```python
from build123d import *

# Parameters (mm, degrees)
SKETCH_1_W          = 49
SKETCH_1_H          = 34.996183206
EXTRUDE_1_DEPTH     = 3
CHAMFER_1_SIZE      = 9.5
FILLET_1_R          = 3
SKETCH_2_R          = 1.65
CUT_EXTRUDE_1_DEPTH = 4


with BuildPart() as part:
    # 草图1 → 凸台-拉伸1 (new body)
    with BuildSketch(Plane.XY):
        Rectangle(SKETCH_1_W, SKETCH_1_H)
    extrude(amount=EXTRUDE_1_DEPTH)

    # 倒角1
    chamfer_1_edges = [part.edges().sort_by_distance(p)[0] for p in [
        (24.5, -17.498091603, 1.5),
        (-24.5, -17.498091603, 1.5),
        (-24.5, 17.498091603, 1.5),
        (24.5, 17.498091603, 1.5),
    ]]
    chamfer(chamfer_1_edges, length=CHAMFER_1_SIZE)

    # 圆角1
    fillet_1_edges = [part.edges().sort_by_distance(p)[0] for p in [
        (-24.5, -7.998091603, 1.5),
        (-24.5, 7.998091603, 1.5),
        (15, 17.498091603, 1.5),
        (-15, 17.498091603, 1.5),
        (15, -17.498091603, 1.5),
        (-15, -17.498091603, 1.5),
        (24.5, 7.998091603, 1.5),
        (24.5, -7.998091603, 1.5),
    ]]
    fillet(fillet_1_edges, radius=FILLET_1_R)

    # 草图2 → 切除-拉伸1 (cut, through all)
    with BuildSketch(Plane.XY.offset(3)):
        with Locations((-21.5, 0)):
            Circle(SKETCH_2_R)
        with Locations((21.5, 0)):
            Circle(SKETCH_2_R)
    extrude(amount=-CUT_EXTRUDE_1_DEPTH, mode=Mode.SUBTRACT)


solid = part.part
```
Verification items for the finished model (mm, model axes). Coordinates: 2 decimals unless noted, no trailing zeros. Write each loop counter-clockwise with the first axis right and the second up, starting at its lowest first coordinate (ties: lowest second). Pieces come first, ordered by that corner, then holes. Notation, with made-up numbers: M -12,-31.75 L 19,-31.75 A19 ccw 19,-7.75 Z; hole C 81.5,58.5 d8. An arc over 180 degrees is marked long. One line per item, written item: value.
Item 1: Scan lines: line 1 along X through (y, z) = (1, 1.7); line 2 along Y through (x, z) = (-20, 2.1); line 3 along Y through (x, z) = (-22, 1.8). Record each from-to range of solid material in increasing order.
Check sheet entries:
line 1: x = -24.5 to -22.81, -20.19 to 20.19, 22.81 to 24.5
line 2: y = -12.5 to -0.69, 0.69 to 12.5
line 3: y = -10.5 to -1.57, 1.57 to 10.5
Item 2: Gauge pin test, flat ends, axial feed: pin 1 Ø2 at (x, y) = (-21.5, 0) entering from -Z; pin 2 Ø6 at (x, y) = (19, 5) entering from -Z. Record the tip position at first contact, or that the pin passes through.
Check sheet entries:
pin 1: passes through
pin 2: stops at z = 0
Item 3: Section check A-A, the plane x = 21.5. Record the boundary of the cut face in (y, z), plus the area to 3 significant figures.
Check sheet entries:
outline: M -11,0 L -1.65,0 L -1.65,3 L -11,3 Z; M 1.65,0 L 11,0 L 11,3 L 1.65,3 Z
area: 56.1 mm^2
Item 4: Mould release check, pull along Y, two halves, no side actions. Record for faces 1 (the cylindrical face through (-14.921, -17.263, 1.521)), 2 (the cylindrical face through (-23.15, 0.07, 1.52)), 3 (the flat face through (19.7, 12.8, 1.5)): pulls with the +Y half, pulls with the -Y half, needs draft (parallel to the pull), parting line crosses it, or undercut.
Check sheet entries:
face 1: pulls with the -Y half
face 2: undercut
face 3: pulls with the +Y half
Item 5: Section check C-C, the plane z = 2. Record the boundary of the cut face in (x, y), plus the area to 3 significant figures.
Check sheet entries:
outline: M -24.5,-6.76 A3 ccw -23.62,-8.88 L -15.88,-16.62 A3 ccw -13.76,-17.5 L 13.76,-17.5 A3 ccw 15.88,-16.62 L 23.62,-8.88 A3 ccw 24.5,-6.76 L 24.5,6.76 A3 ccw 23.62,8.88 L 15.88,16.62 A3 ccw 13.76,17.5 L -13.76,17.5 A3 ccw -15.88,16.62 L -23.62,8.88 A3 ccw -24.5,6.76 Z; hole C -21.5,0 d3.3; hole C 21.5,0 d3.3
area: 1,520 mm^2
Item 6: Section check B-B, the plane y = 0. Record the boundary of the cut face in (x, z).
Check sheet entries:
outline: M -24.5,0 L -23.15,0 L -23.15,3 L -24.5,3 Z; M -19.85,0 L 19.85,0 L 19.85,3 L -19.85,3 Z; M 23.15,0 L 24.5,0 L 24.5,3 L 23.15,3 Z
